Geometry check sheet. Reference: the model listing, model coordinates, mm. A direction names the side the tool comes from. Give positions to 0.01 mm unless a question says otherwise; leave off trailing zeros. Loops run counter-clockwise (first coordinate to the right, second up) from the corner with the lowest first, then second, coordinate; pieces in that order, holes last. Notation, with made-up numbers: (16, 82) -> (73, 82) arc R25 cw to (73, 104) -> close; hole circle Ø10 at (-3, -5.5). An arc over 180 degrees is marked (long way). Write item = value, one per line. Start each with the question number.
```python
from build123d import *

# Parameters (mm, degrees)
SKETCH_1_W          = 300
SKETCH_1_H          = 40
EXTRUDE_1_DEPTH     = 10
CUT_EXTRUDE_1_REACH = 12


with BuildPart() as part:
    # Эскиз1 → Бобышка-Вытянуть1 (new body)
    with BuildSketch(Plane(origin=(0, 0, 0), x_dir=(1, 0, 0), z_dir=(0, 1, 0))):
        with Locations((150, 20)):
            Rectangle(SKETCH_1_W, SKETCH_1_H)
    extrude(amount=EXTRUDE_1_DEPTH)

    # Эскиз2 → Вырез-Вытянуть1 (cut, up to next)
    with BuildSketch(Plane(origin=(0, 10, 0), x_dir=(1, 0, 0), z_dir=(0, 1, 0)), mode=Mode.PRIVATE) as cut_extrude_1_sk1:
        with BuildLine():
            Line((95, 9.95), (274.721446052, 9.953861055))
            ThreePointArc((274.721446052, 9.953861055), (285.05, 20), (274.721446052, 30.046138945))
            Line((274.721446052, 30.046138945), (95, 30.05))
            ThreePointArc((95, 30.05), (84.95, 20), (95, 9.95))
        make_face()
    cut_extrude_1_tool1 = extrude(cut_extrude_1_sk1.sketch, amount=-CUT_EXTRUDE_1_REACH, mode=Mode.PRIVATE) & part.part
    add(cut_extrude_1_tool1.solids().sort_by_distance((184.994726, 10, -20))[0], mode=Mode.SUBTRACT)


solid = part.part
```
1) Thickness scan on line 1 (Z direction, x = 159, y = 7); line 2 (X direction, y = 2.25, z = -19.5); line 3 (X direction, y = 7.5, z = -12). Record the ranges inside material, lowest first.
2) Section check B-B (y = 1.5). Enter the section's corners in (x, z), plus the area to 3 significant figures.
3) Section check C-C (x = 128.5). Enter the section's corners in (y, z).
4) Draft check along Z on faces 3 (the flat face through (0, 5, -20)), 4 (the flat face through (148, 5, 0)), 5 (the cylindrical face through (84.952, 5.07, -20.221)). Enter one of: released by +Z, released by -Z, zero draft, split by the parting line, or undercut.
5) Tool access check on faces 1 (the cylindrical face through (285.047, 5.07, -19.775)), 2 (the flat face through (115, 0, -34)). Record the directions out of +Z, -Z, +X, -X, +Y, -Y that give a thin tool (end or side, any length) a straight path to the whole face; none if there is none.
6) Section check A-A (z = -20). Enter the section's corners in (x, y), plus the area to 3 significant figures.
7) Depth check by flat-ended pin: pin 1 Ø1.5 at (x, z) = (184, -4.5) entering from -Y; pin 2 Ø6 at (x, z) = (179, -25) entering from +Y. Enter the tip coordinate at first touch or a pass-through.
Check result:
q1.line_1 = -40 to -30.05, -9.95 to 0
q1.line_2 = 0 to 84.96, 285.04 to 300
q1.line_3 = 0 to 88.92, 281.08 to 300
q2.outline = (0, -40) -> (300, -40) -> (300, 0) -> (0, 0) -> close; hole (95, -30.05) -> (274.72, -30.05) arc R10.05 ccw (long way) to (274.72, -9.95) -> (95, -9.95) arc R10.05 ccw to start
q2.area = 8,070 mm2
q3.outline = (0, -40) -> (10, -40) -> (10, -30.05) -> (0, -30.05) -> close; (0, -9.95) -> (10, -9.95) -> (10, 0) -> (0, 0) -> close
q4.face_3 = zero draft
q4.face_4 = released by +Z
q4.face_5 = undercut
q5.face_1 = +Y, -Y
q5.face_2 = +Z, -Z, +X, -X, -Y
q6.outline = (0, 0) -> (84.95, 0) -> (84.95, 10) -> (0, 10) -> close; (285.05, 0) -> (300, 0) -> (300, 10) -> (285.05, 10) -> close
q6.area = 999 mm2
q7.pin_1 = 0
q7.pin_2 = through
